Input: part model. Units: mm. Frame: model coordinates. A direction names the side the tool comes from. Coordinates: 2 decimals unless noted, no trailing zeros. Loops run counter-clockwise (first coordinate to the right, second up) from the corner with the lowest first, then second, coordinate; pieces in that order, holes last.
```python
from build123d import *

# Parameters (mm, degrees)
SKETCH1_W           = 418.07892
SKETCH1_H           = 415.925
BOSS_EXTRUDE1_DEPTH = 12.7
SKETCH2_W           = 418.07892
SKETCH2_H           = 107.95
BOSS_EXTRUDE2_DEPTH = 12.7
SKETCH3_W           = 418.07892
SKETCH3_H           = 12.923123126
BOSS_EXTRUDE3_DEPTH = 12.7
BOSS_EXTRUDE4_DEPTH = 12.7
CHAMFER1_SIZE       = 304.8
CHAMFER1_SIZE_2     = 19.05


with BuildPart() as part:
    # Sketch1 → Boss-Extrude1 (new body)
    with BuildSketch(Plane.XY):
        with Locations((0, -5261.217030575)):
            Rectangle(SKETCH1_W, SKETCH1_H)
    extrude(amount=BOSS_EXTRUDE1_DEPTH)

    # Sketch2 → Boss-Extrude2 (add, through all)
    with BuildSketch(Plane(origin=(0, 0, 0), x_dir=(-1, 0, 0), z_dir=(0, 0, -1))):
        with Locations((0, -5523.154530575)):
            Rectangle(SKETCH2_W, SKETCH2_H)
    extrude(amount=-BOSS_EXTRUDE2_DEPTH)

    # Sketch3 → Boss-Extrude3 (add, through all)
    with BuildSketch(Plane(origin=(0, 0, 0), x_dir=(-1, 0, 0), z_dir=(0, 0, -1))):
        with Locations((0, -5046.792969012)):
            Rectangle(SKETCH3_W, SKETCH3_H)
    extrude(amount=-BOSS_EXTRUDE3_DEPTH)

    # Sketch4 → Boss-Extrude4 (add, through all)
    with BuildSketch(Plane(origin=(0, 0, 0), x_dir=(-1, 0, 0), z_dir=(0, 0, -1))):
        Polygon((209.038766336, -5462.805770365), (228.088766336, -5462.805770365), (228.088766336, -5577.129530575), (209.03946, -5577.129530575), align=None)
        Polygon((-209.03946, -5577.129530575), (-209.038766336, -5462.805770365), (-228.088766336, -5462.805770365), (-228.088766336, -5577.129530575), align=None)
    extrude(amount=-BOSS_EXTRUDE4_DEPTH)

    # Chamfer1
    # the kernel refuses this chamfer: 304.8, 19.05 mm, written as the material it adds along each edge
    with BuildSketch(Plane(origin=(-209.03946, -5462.805770365, 0), x_dir=(0.002399337658707147, 0.9999971215852571, 0), z_dir=(0, 0, 1))) as chamfer1_piece_1_section:
        Polygon((CHAMFER1_SIZE * 0.999997121585, CHAMFER1_SIZE * 0.00239933765871), (-CHAMFER1_SIZE_2 * 0.00239933765871, CHAMFER1_SIZE_2 * 0.999997121585), (0, 0), align=None)
    chamfer1_piece_1 = extrude(amount=12.7, mode=Mode.PRIVATE)
    chamfer1_piece_1 = split(chamfer1_piece_1, bisect_by=Plane(origin=(-228.088766336, -5341.135021574, 6.35), z_dir=(1, 0, 0)), keep=Keep.TOP, mode=Mode.PRIVATE)
    add(chamfer1_piece_1)
    with BuildSketch(Plane(origin=(209.03946, -5462.805770365, 0), x_dir=(0.8520963193143735, -0.5233850041899339, 0), z_dir=(0, 0, 1))) as chamfer1_piece_2_section:
        Polygon((CHAMFER1_SIZE_2 * 0.852096319314, CHAMFER1_SIZE_2 * 0.52338500419), (-CHAMFER1_SIZE * 0.52338500419, CHAMFER1_SIZE * 0.852096319314), (0, 0), align=None)
    chamfer1_piece_2 = extrude(amount=12.7, mode=Mode.PRIVATE)
    chamfer1_piece_2 = split(chamfer1_piece_2, bisect_by=Plane(origin=(228.088766336, -5341.135021574, 6.35), z_dir=(-1, 0, 0)), keep=Keep.TOP, mode=Mode.PRIVATE)
    add(chamfer1_piece_2)


solid = part.part
```
Item 1: Section query A-A (z = 6.75). Output: boundary loops of the cut face in (x, y).
Result:
outline: (-228.09, -5577.13) - (228.09, -5577.13) - (228.09, -5462.79) - (209.04, -5158.01) - (209.04, -5040.33) - (-209.04, -5040.33) - (-209.04, -5158.01) - (-228.09, -5462.79) - close
Item 2: Contact query for flat-ended pins moving along their axis: P1, Ø4, axis at y = -5128.5, z = 5, coming from the -X side; P2, Ø6, axis at y = -5410.5, z = 7.5, coming from the -X side; P3, Ø4, axis at y = -5084.5, z = 8, coming from the +X side. Output: stop coordinate, or through.
Result:
P1: stops at x = -209.04
P2: stops at x = -225.01
P3: stops at x = 209.04
Item 3: Reachability of faces 1 (the face through (-209.039, -5100, 6)), 2 (the face through (-228.089, -5521, 6)), 3 (the face through (209.039, -5100, 6)) from +Z, -Z, +X, -X, +Y, -Y: full face, straight path, thin tool, end or side. Return the list, or none.
Result:
face 1: +Z, -Z, -X, +Y
face 2: +Z, -Z, -X, +Y, -Y
face 3: +Z, -Z, +X, +Y
Item 4: Line query: L1, parallel to X at y = -5136, z = 12.25; L2, parallel to X at y = -5237, z = 2.25. Output: solid intervals per line, ascending.
Result:
L1: x = -209.04 to 209.04
L2: x = -213.98 to 213.98
Item 5: Section query C-C (y = -5255). Output: boundary loops of the cut face in (x, z), then the cut area to 3 significant figures.
Result:
outline: (-215.1, 0) - (215.1, 0) - (215.1, 12.7) - (-215.1, 12.7) - close
area: 5,460 mm2
Item 6: Section query B-B (y = -5150). Output: boundary loops of the cut face in (x, z).
Result:
outline: (-209.04, 0) - (209.04, 0) - (209.04, 12.7) - (-209.04, 12.7) - close
